Geometry: final body of the model. Coordinates: model frame, mm. Face numbers are marked on the shaded views. A direction names the side the tool comes from. Coordinates: 2 decimals unless noted, no trailing zeros. Order: outer loops, then holes, each group sorted by start corner. A loop starts at its lowest first (then second) coordinate and runs counter-clockwise, first axis right, second up. Notation, with made-up numbers: M -5.75,43.25 L 40.25,43.25 A23 ccw 40.25,67.25 Z; hole C -16,-2.75 d11. An arc over 180 degrees is marked long. Write item = value, one per line. Start each with the question number.
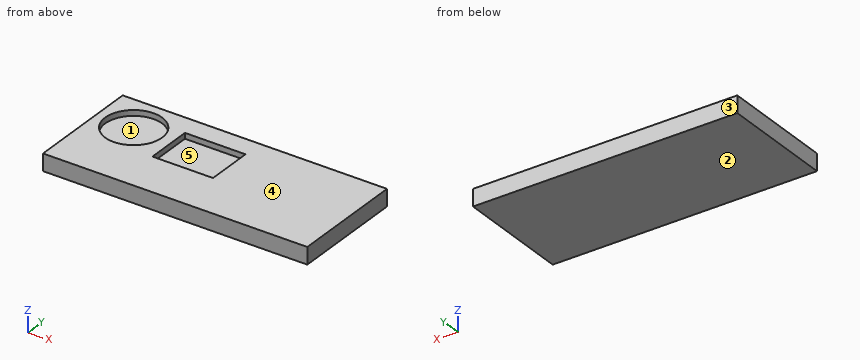
```python
from build123d import *

# Parameters (mm, degrees)
F0_W     = 235.307321
F0_H     = 101.85823
F1_DEPTH = 15
F2_R     = 25.336602
F3_DEPTH = 5
F4_W     = 53.954252
F4_H     = 41.550964
F5_DEPTH = 5


with BuildPart() as f1:
    # F0 (on Top) → F1 (new body)
    with BuildSketch(Plane.XY):
        with Locations((117.653661, 52.72521)):
            Rectangle(F0_W, F0_H)
    extrude(amount=F1_DEPTH)

    # F2 (on face) → F3 (cut)
    with BuildSketch(Plane.XY.offset(15)):
        with Locations((33.09346, 70.193075)):
            Circle(F2_R)
    extrude(amount=-F3_DEPTH, mode=Mode.SUBTRACT)

    # F4 (on face) → F5 (cut)
    with BuildSketch(Plane.XY.offset(15)):
        with Locations((95.118355, 64.582877)):
            Rectangle(F4_W, F4_H)
    extrude(amount=-F5_DEPTH, mode=Mode.SUBTRACT)


solid = f1.part
```
Item 1: Section query A-A on x = 98. Output: boundary loops of the cut face in (y, z), and give its area (3 significant figures).
Item 2: Draft query along Y for the marked faces 1, 2 and 3. Return one class per face: pulls with the +Y half, pulls with the -Y half, needs draft (parallel to the pull), parting line crosses it, or undercut.
Item 3: Section query B-B on y = 67. Output: boundary loops of the cut face in (x, z).
Item 4: Section query C-C on x = 22.5. Output: boundary loops of the cut face in (y, z).
Item 5: Reachability of the marked faces 4 and 5 from +Z, -Z, +X, -X, +Y, -Y: full face, straight path, thin tool, end or side. Return the list, or none.
Item 6: Material intervals for probe 1 along Y at (x, z) = (116.5, 12); probe 2 along Y at (x, z) = (26.5, 14.25); probe 3 along Z at (x, y) = (38.5, 91.5), sorted ascending. Write a range as [from, to].
Ans:
q1.outline = M 1.8,0 L 103.65,0 L 103.65,15 L 85.36,15 L 85.36,10 L 43.81,10 L 43.81,15 L 1.8,15 Z
q1.area = 1,320 mm^2
q2.face_1 = undercut
q2.face_2 = needs draft
q2.face_3 = pulls with the +Y half
q3.outline = M 0,0 L 235.31,0 L 235.31,15 L 122.1,15 L 122.1,10 L 68.14,10 L 68.14,15 L 58.23,15 L 58.23,10 L 7.96,10 L 7.96,15 L 0,15 Z
q4.outline = M 1.8,0 L 103.65,0 L 103.65,15 L 93.21,15 L 93.21,10 L 47.18,10 L 47.18,15 L 1.8,15 Z
q5.face_4 = +Z, +X, -X, +Y, -Y
q5.face_5 = +Z
q6.probe_1 = [1.8, 43.81], [85.36, 103.65]
q6.probe_2 = [1.8, 45.73], [94.66, 103.65]
q6.probe_3 = [0, 10]
